```python
from build123d import *

# Parameters (mm, degrees)
SKETCH_1_W          = 36
SKETCH_1_H          = 42
EXTRUDE_1_DEPTH     = 2
SKETCH_2_W          = 32
SKETCH_2_H          = 2.5
EXTRUDE_2_DEPTH     = 9.5
SKETCH_3_W          = 3
SKETCH_3_H          = 39.5
CUT_EXTRUDE_1_DEPTH = 1
SKETCH_4_R          = 2
SKETCH_4_R_2        = 1.1
EXTRUDE_3_DEPTH     = 4
SKETCH_4_2_R        = 2
EXTRUDE_4_DEPTH     = 1
EXTRUDE_5_DEPTH     = 4
EXTRUDE_6_DEPTH     = 4
SKETCH_8_R          = 2.5
EXTRUDE_7_DEPTH     = 4
SKETCH_9_W          = 9.5
SKETCH_9_H          = 1.5
EXTRUDE_8_DEPTH     = 4


with BuildPart() as part:
    # 草图1 → 凸台-拉伸1 (new body)
    with BuildSketch(Plane.XY):
        with Locations((-3, 0)):
            Rectangle(SKETCH_1_W, SKETCH_1_H)
    extrude(amount=EXTRUDE_1_DEPTH)

    # 草图2 → 凸台-拉伸2 (add)
    with BuildSketch(Plane(origin=(0, 0, 0), x_dir=(-1, 0, 0), z_dir=(0, 0, -1))):
        with Locations((5, 19.75)):
            Rectangle(SKETCH_2_W, SKETCH_2_H)
        with Locations((5, -19.75)):
            Rectangle(SKETCH_2_W, SKETCH_2_H)
    extrude(amount=EXTRUDE_2_DEPTH)

    # 草图3 → 切除-拉伸1 (cut)
    with BuildSketch(Plane(origin=(0, 0, 0), x_dir=(-1, 0, 0), z_dir=(0, 0, -1))):
        with Locations((-12.5, 0)):
            Rectangle(SKETCH_3_W, SKETCH_3_H)
    extrude(amount=-CUT_EXTRUDE_1_DEPTH, mode=Mode.SUBTRACT)

    # 草图4 → 凸台-拉伸3 (add)
    with BuildSketch(Plane(origin=(0, 0, 0), x_dir=(-1, 0, 0), z_dir=(0, 0, -1))):
        with Locations((11, 15.5)):
            Circle(SKETCH_4_R)
        with Locations((11, 15.5)):
            Circle(SKETCH_4_R_2, mode=Mode.SUBTRACT)
        with Locations((-11, -15.5)):
            Circle(SKETCH_4_R)
        with Locations((-11, -15.5)):
            Circle(SKETCH_4_R_2, mode=Mode.SUBTRACT)
    extrude(amount=EXTRUDE_3_DEPTH)

    # 草图4<2> → 凸台-拉伸4 (add)
    with BuildSketch(Plane(origin=(0, 0, 0), x_dir=(-1, 0, 0), z_dir=(0, 0, -1))):
        with Locations((-11, -15.5)):
            Circle(SKETCH_4_2_R)
    extrude(amount=-EXTRUDE_4_DEPTH)

    # 草图5 → 凸台-拉伸5 (add)
    with BuildSketch(Plane(origin=(0, 0, 0), x_dir=(-1, 0, 0), z_dir=(0, 0, -1))):
        Polygon((9, 15.5), (9, 18.5), (13, 18.5), (13, 15.5), (11, 17.5), align=None)
    extrude(amount=EXTRUDE_5_DEPTH)

    # 草图6 → 凸台-拉伸6 (add)
    with BuildSketch(Plane(origin=(0, 0, 0), x_dir=(-1, 0, 0), z_dir=(0, 0, -1))):
        Polygon((-11, -17.5), (-11, -18.5), (-9, -18.5), (-9, -15.5), align=None)
    extrude(amount=EXTRUDE_6_DEPTH)

    # 草图8 → 凸台-拉伸7 (add)
    with BuildSketch(Plane(origin=(0, 0, 0), x_dir=(-1, 0, 0), z_dir=(0, 0, -1))):
        with Locations((7.5, -12.5)):
            Circle(SKETCH_8_R)
        with Locations((-7.5, 12.5)):
            Circle(SKETCH_8_R)
    extrude(amount=EXTRUDE_7_DEPTH)

    # 草图9 → 凸台-拉伸8 (add)
    with BuildSketch(Plane.ZY.offset(21)):
        with Locations((-4.75, -17.75)):
            Rectangle(SKETCH_9_W, SKETCH_9_H)
        with Locations((-4.75, 17.75)):
            Rectangle(SKETCH_9_W, SKETCH_9_H)
    extrude(amount=-EXTRUDE_8_DEPTH)


solid = part.part
```
Verification items for the finished model (mm, model axes). A direction names the side the tool comes from. Give positions to 0.01 mm unless a question says otherwise; leave off trailing zeros. Write each loop counter-clockwise with the first axis right and the second up, starting at its lowest first coordinate (ties: lowest second). Pieces come first, ordered by that corner, then holes. Notation, with made-up numbers: (-6, -32) - (15, -32) arc R27 ccw to (15, -12) - close; hole circle Ø9 at (-25.75, 61). An arc over 180 degrees is marked (long way). Put each result on its own line as item: value.
Q1. Section check B-B on x = 7.5. Record the cut outline in (y, z), and give its area (4 significant figures).
Result:
outline: (-21, -9.5) - (-18.5, -9.5) - (-18.5, 0) - (10, 0) - (10, -4) - (15, -4) - (15, 0) - (18.5, 0) - (18.5, -9.5) - (21, -9.5) - (21, 2) - (-21, 2) - close
area: 151.5 mm2
Q2. Set-up check for faces 1 (the face through (-17, 18, -5)), 2 (the face through (15, 0, 1)), 3 (the face through (-3, -21, -4)), 4 (the face through (-9, 17, -2)), 5 (the face through (-19, -17, -5)): record each of +Z, -Z, +X, -X, +Y, -Y from which the full face is reachable in a straight line by a thin tool's end or side.
Result:
face 1: -Z
face 2: +Z, -Z, +X, +Y, -Y
face 3: +Z, -Z, +X, -X, -Y
face 4: -Z, +X
face 5: -Z, -X
Q3. Section check D-D on x = -11. Record the cut outline in (y, z), and give its area (3 significant figures).
Result:
outline: (-21, -9.5) - (-18.5, -9.5) - (-18.5, 0) - (13.5, 0) - (13.5, -4) - (14.4, -4) - (14.4, 0) - (16.6, 0) - (16.6, -4) - (18.5, -4) - (18.5, -9.5) - (21, -9.5) - (21, 2) - (-21, 2) - close
area: 143 mm2
Q4. Section check A-A on z = -0.5. Record the cut outline in (x, y).
Result:
outline: (-21, -21) - (11, -21) - (11, -17.5) arc R2 ccw (long way) to (9, -15.5) - (9, -18.5) - (-17, -18.5) - (-17, -17) - (-21, -17) - close; (-21, 17) - (-17, 17) - (-17, 18.5) - (-13, 18.5) - (-13, 15.5) arc R2 ccw to (-9, 15.5) - (-9, 18.5) - (11, 18.5) - (11, 21) - (-21, 21) - close; circle Ø5 at (-7.5, -12.5); circle Ø5 at (7.5, 12.5); hole circle Ø2.2 at (-11, 15.5); hole circle Ø2.2 at (11, -15.5)
Q5. Depth check by flat-ended pin: P1, Ø3.5, axis at x = 12, y = 6, coming from the -Z side; P2, Ø1.5, axis at y = 17.5, z = -1.5, coming from the +X side; P3, Ø4, axis at y = 14.5, z = -1.5, coming from the +X side; P4, Ø1.2, axis at x = 10, y = -16, coming from the -Z side. Enter the tip coordinate at first touch or a pass-through.
Result:
P1: z = 0
P2: x = -9
P3: x = 15
P4: z = -4
Q6. Mould release check, pull along Y, two halves, no side actions. Record for faces 6 (the face through (-3, 21, -4)), 7 (the face through (12.5, -19.75, 0.5)), 8 (the face through (14.3, 0.1, 0)): released by +Y, released by -Y, zero draft, split by the parting line, or undercut.
Result:
face 6: released by +Y
face 7: undercut
face 8: zero draft
Q7. Scan lines: probe 1 along Y at (x, z) = (-11, -2.7); probe 2 along Y at (x, z) = (-8, -4.5); probe 3 along Y at (x, z) = (-18, -5.25). Record each from-to range of solid material in increasing order. Write a range as from..to.
Result:
probe 1: -21..-18.5, 13.5..14.4, 16.6..21
probe 2: -21..-18.5, 18.5..21
probe 3: -21..-17, 17..21
Q8. Section check C-C on y = -7. Record the cut outline in (x, z), and give its area (3 significant figures).
Result:
outline: (-21, 0) - (11, 0) - (11, 1) - (14, 1) - (14, 0) - (15, 0) - (15, 2) - (-21, 2) - close
area: 69.0 mm2
